from build123d import *

# Parameters (mm, degrees)
SKETCH1_W                                           = 107
SKETCH1_H                                           = 26
BOSS_EXTRUDE1_DEPTH                                 = 8
SKETCH2_W                                           = 1
SKETCH2_H                                           = 7.5
SKETCH2_W_2                                         = 6
SKETCH2_H_2                                         = 6.5
CUT_EXTRUDE1_DEPTH                                  = 111.403804282
FILLET1_R                                           = 0.5
CSK_FOR_M2_COUNTERSUNK_FLAT_HEAD_SCREW1_D           = 2.4
CSK_FOR_M2_COUNTERSUNK_FLAT_HEAD_SCREW1_DEPTH       = 15
CSK_FOR_M2_COUNTERSUNK_FLAT_HEAD_SCREW1_CSINK_D     = 4.4
CSK_FOR_M2_COUNTERSUNK_FLAT_HEAD_SCREW1_CSINK_ANGLE = 90
CSK_FOR_M2_COUNTERSUNK_FLAT_HEAD_SCREW1_TIP         = 0.721032743
SKETCH14_W                                          = 97
SKETCH14_H                                          = 24
CUT_EXTRUDE7_DEPTH                                  = 111.403804282
SKETCH14_3_W                                        = 97
SKETCH14_3_H                                        = 24
BOSS_EXTRUDE3_DEPTH                                 = 1
SKETCH18_W                                          = 97
SKETCH18_H                                          = 24
CUT_EXTRUDE8_DEPTH                                  = 111.403804282
SKETCH20_W                                          = 97
SKETCH20_H                                          = 24
SKETCH20_W_2                                        = 93
SKETCH20_H_2                                        = 20
BOSS_EXTRUDE4_DEPTH                                 = 8
SKETCH20_2_W                                        = 97
SKETCH20_2_H                                        = 24
SKETCH20_2_W_2                                      = 93
SKETCH20_2_H_2                                      = 20
CUT_EXTRUDE9_DEPTH                                  = 3
SKETCH21_W                                          = 52
SKETCH21_H                                          = 2
BOSS_EXTRUDE5_DEPTH                                 = 5
SKETCH22_W                                          = 52
SKETCH22_H                                          = 2
BOSS_EXTRUDE6_DEPTH                                 = 5
SKETCH23_W                                          = 0.5
SKETCH23_H                                          = 16.612240618
CUT_EXTRUDE10_DEPTH                                 = 111.403804282
BOSS_EXTRUDE7_REACH                                 = 111.249
SKETCH25_W                                          = 2
SKETCH25_H                                          = 5
CUT_EXTRUDE11_REACH                                 = 64.258
SKETCH26_W                                          = 10
SKETCH26_H                                          = 2
SKETCH27_W                                          = 97
SKETCH27_H                                          = 24
BOSS_EXTRUDE8_DEPTH                                 = 3
SKETCH29_W                                          = 20
SKETCH29_H                                          = 5
CUT_EXTRUDE12_DEPTH                                 = 54


with BuildPart() as part:
    # Sketch1 → Boss-Extrude1 (new body)
    with BuildSketch(Plane(origin=(0, 0, 0), x_dir=(1, 0, 0), z_dir=(0, 1, 0))):
        with Locations((53.5, -13)):
            Rectangle(SKETCH1_W, SKETCH1_H)
    extrude(amount=BOSS_EXTRUDE1_DEPTH)

    # Sketch2 → Cut-Extrude1 (cut, through all)
    with BuildSketch(Plane.XY.offset(26)):
        with Locations((106.5, 4.25)):
            Rectangle(SKETCH2_W, SKETCH2_H)
        with Locations((3, 4.75)):
            Rectangle(SKETCH2_W_2, SKETCH2_H_2)
    extrude(amount=-CUT_EXTRUDE1_DEPTH, mode=Mode.SUBTRACT)

    # Fillet1
    fillet1_edges = [part.edges().sort_by_distance(p)[0] for p in [
        (106, 8, 13),
        (0, 1.5, 13),
        (6, 8, 13),
    ]]
    fillet(fillet1_edges, radius=FILLET1_R)

    # CSK for M2 Countersunk Flat Head Screw1
    with Locations(Plane(origin=(3, 1.5, 13), x_dir=(1, 0, 0), z_dir=(0, 1, 0))):
        with Locations((0, 0)):
            CounterSinkHole(CSK_FOR_M2_COUNTERSUNK_FLAT_HEAD_SCREW1_D / 2, CSK_FOR_M2_COUNTERSUNK_FLAT_HEAD_SCREW1_CSINK_D / 2, depth=CSK_FOR_M2_COUNTERSUNK_FLAT_HEAD_SCREW1_DEPTH, counter_sink_angle=CSK_FOR_M2_COUNTERSUNK_FLAT_HEAD_SCREW1_CSINK_ANGLE)
            with Locations((0, 0, -(CSK_FOR_M2_COUNTERSUNK_FLAT_HEAD_SCREW1_DEPTH + CSK_FOR_M2_COUNTERSUNK_FLAT_HEAD_SCREW1_TIP / 2))):  # 118° drill point
                Cone(0, CSK_FOR_M2_COUNTERSUNK_FLAT_HEAD_SCREW1_D / 2, CSK_FOR_M2_COUNTERSUNK_FLAT_HEAD_SCREW1_TIP, mode=Mode.SUBTRACT)

    # Sketch14 → Cut-Extrude7 (cut, through all)
    with BuildSketch(Plane(origin=(0, 8, 0), x_dir=(1, 0, 0), z_dir=(0, 1, 0))):
        with Locations((56, -13)):
            Rectangle(SKETCH14_W, SKETCH14_H)
    extrude(amount=-CUT_EXTRUDE7_DEPTH, mode=Mode.SUBTRACT)

    # Sketch14<3> → Boss-Extrude3 (add)
    with BuildSketch(Plane(origin=(0, 8, 0), x_dir=(1, 0, 0), z_dir=(0, 1, 0))):
        with Locations((56, -13)):
            Rectangle(SKETCH14_3_W, SKETCH14_3_H)
    extrude(amount=-BOSS_EXTRUDE3_DEPTH)

    # Sketch18 → Cut-Extrude8 (cut, through all)
    with BuildSketch(Plane(origin=(0, 0, 0), x_dir=(1, 0, 0), z_dir=(0, 1, 0))):
        with Locations((56, -13)):
            Rectangle(SKETCH18_W, SKETCH18_H)
    extrude(amount=CUT_EXTRUDE8_DEPTH, mode=Mode.SUBTRACT)

    # Sketch20 → Boss-Extrude4 (add)
    with BuildSketch(Plane(origin=(0, 8, 0), x_dir=(1, 0, 0), z_dir=(0, 1, 0))):
        with Locations((56, -13)):
            Rectangle(SKETCH20_W, SKETCH20_H)
        with Locations((56, -13)):
            Rectangle(SKETCH20_W_2, SKETCH20_H_2, mode=Mode.SUBTRACT)
    extrude(amount=-BOSS_EXTRUDE4_DEPTH)

    # Sketch20<2> → Cut-Extrude9 (cut)
    with BuildSketch(Plane(origin=(0, 8, 0), x_dir=(1, 0, 0), z_dir=(0, 1, 0))):
        with Locations((56, -13)):
            Rectangle(SKETCH20_2_W, SKETCH20_2_H)
        with Locations((56, -13)):
            Rectangle(SKETCH20_2_W_2, SKETCH20_2_H_2, mode=Mode.SUBTRACT)
    extrude(amount=-CUT_EXTRUDE9_DEPTH, mode=Mode.SUBTRACT)

    # Sketch21 → Boss-Extrude5 (add)
    with BuildSketch(Plane.XY.offset(3)):
        with Locations((76.5, 1)):
            Rectangle(SKETCH21_W, SKETCH21_H)
    extrude(amount=BOSS_EXTRUDE5_DEPTH)

    # Sketch22 → Boss-Extrude6 (add)
    with BuildSketch(Plane(origin=(0, 0, 23), x_dir=(-1, 0, 0), z_dir=(0, 0, -1))):
        with Locations((-76.5, 1)):
            Rectangle(SKETCH22_W, SKETCH22_H)
    extrude(amount=BOSS_EXTRUDE6_DEPTH)

    # Sketch23 → Cut-Extrude10 (cut, through all)
    with BuildSketch(Plane.XY.offset(26)):
        with Locations((106.75, 8.306120309)):
            Rectangle(SKETCH23_W, SKETCH23_H)
    extrude(amount=-CUT_EXTRUDE10_DEPTH, mode=Mode.SUBTRACT)

    # Sketch25 → Boss-Extrude7 (add, up to next)
    with BuildSketch(Plane(origin=(0, 0, 23), x_dir=(-1, 0, 0), z_dir=(0, 0, -1)), mode=Mode.PRIVATE) as boss_extrude7_sk1:
        with Locations((-49.5, 2.5)):
            Rectangle(SKETCH25_W, SKETCH25_H)
    boss_extrude7_tool1 = extrude(boss_extrude7_sk1.sketch, amount=BOSS_EXTRUDE7_REACH, mode=Mode.PRIVATE) - part.part
    add(boss_extrude7_tool1.solids().sort_by_distance((49.5, 2.5, 23))[0])

    # Sketch26 → Cut-Extrude11 (cut, up to next)
    with BuildSketch(Plane(origin=(50.5, 0, 0), x_dir=(0, 0, -1), z_dir=(1, 0, 0)), mode=Mode.PRIVATE) as cut_extrude11_sk1:
        with Locations((-13, 1)):
            Rectangle(SKETCH26_W, SKETCH26_H)
    cut_extrude11_tool1 = extrude(cut_extrude11_sk1.sketch, amount=-CUT_EXTRUDE11_REACH, mode=Mode.PRIVATE) & part.part
    add(cut_extrude11_tool1.solids().sort_by_distance((50.5, 1, 13))[0], mode=Mode.SUBTRACT)

    # Sketch27 → Boss-Extrude8 (add)
    with BuildSketch(Plane(origin=(0, 5, 0), x_dir=(1, 0, 0), z_dir=(0, 1, 0))):
        with Locations((56, -13)):
            Rectangle(SKETCH27_W, SKETCH27_H)
    extrude(amount=BOSS_EXTRUDE8_DEPTH)

    # Sketch29 → Cut-Extrude12 (cut)
    with BuildSketch(Plane.ZY.offset(-48.5)):
        with Locations((13, 2.5)):
            Rectangle(SKETCH29_W, SKETCH29_H)
    extrude(amount=-CUT_EXTRUDE12_DEPTH, mode=Mode.SUBTRACT)


solid = part.part
Here's how the part is built. I have some questions about the finished solid (model axes, mm). A direction names the side the tool comes from. Round coordinates to 2 decimals unless told otherwise and drop trailing zeros. Order: outer loops, then holes, each group sorted by start corner. A loop starts at its lowest first (then second) coordinate and runs counter-clockwise, first axis right, second up. Notation, with made-up numbers: M 86.25,88.25 L 91.25,88.25 A14 ccw 91.25,111.25 Z; hole C 53,41.5 d11. An arc over 180 degrees is marked long. One line per question, with ' | ' between items.
1) We'd pull the mould along X, two halves only. Please class faces 4 (the flat face through (6, 4, 13)), 5 (the flat face through (50, 0, 2)), 6 (the flat face through (55, 5, 13)): released by +X, released by -X, zero draft, split by the parting line, or undercut.
Checked values:
face 4: released by -X | face 5: zero draft | face 6: undercut
2) I need wall thicknesses on line 1 (Z direction, x = 98, y = 4.75); line 2 (X direction, y = 4, z = 7); line 3 (X direction, y = 0.35, z = 13). Which ranges of each line are inside material? Lowest first, please.
Checked values:
line 1: z = 0 to 3, 23 to 26 | line 2: x = 6 to 9.5, 102.5 to 106 | line 3: x = 0 to 1.8, 4.2 to 9.5, 102.5 to 106.5
3) On a 3-axis mill with a long thin cutter (end or side, diameter ignored), from which of +Z, -Z, +X, -X, +Y, -Y can I reach the whole of each face in a straight line? I mean faces 1 (the flat face through (5.7, 1.5, 13.2)), 2 (the flat face through (9.5, 3, 13)), 3 (the flat face through (106, 4, 13)). Say none if no direction works.
Checked values:
face 1: +Z, -Z, -X, +Y | face 2: -Y | face 3: +Z, -Z, +X, +Y
4) Imagine slicing it at D-D, the plane x = 99. Write out the boundary of the cut face in (y, z), plus the area to 3 significant figures.
Checked values:
outline: M 0,0 L 8,0 L 8,26 L 0,26 L 0,23 L 5,23 L 5,3 L 0,3 Z | area: 108 mm²
5) Imagine slicing it at A-A, the plane z = 13. Write out the boundary of the cut face in (x, y).
Checked values:
outline: M 0,0 L 1.8,0 L 1.8,0.5 L 0.8,1.5 L 0.5,1.5 A0.5 ccw 0,1 Z; M 4.2,0 L 9.5,0 L 9.5,5 L 102.5,5 L 102.5,0 L 106.5,0 L 106.5,0.5 L 106,0.5 L 106,7.5 A0.5 ccw 105.5,8 L 6.5,8 A0.5 ccw 6,7.5 L 6,1.5 L 5.2,1.5 L 4.2,0.5 Z
6) Imagine slicing it at B-B, the plane x = 3. Write out the boundary of the cut face in (y, z), plus the area to 3 significant figures.
Checked values:
outline: M 0,0 L 1.5,0 L 1.5,10.8 L 0.5,11.8 L 0,11.8 Z; M 0,14.2 L 0.5,14.2 L 1.5,15.2 L 1.5,26 L 0,26 Z | area: 34.4 mm²
7) I'm going to push flat-ended pins straight in: pin 1 Ø4 at (y, z) = (1.5, 11) entering from -X; pin 2 Ø3.5 at (y, z) = (3, 7.5) entering from +X; pin 3 Ø2 at (y, z) = (6.5, 23.5) entering from -X; pin 4 Ø2 at (x, z) = (14.5, 10.5) entering from -Y. Where does each tip first touch, or does it pass through?
Checked values:
pin 1: stops at x = 0 | pin 2: stops at x = 106 | pin 3: stops at x = 6 | pin 4: stops at y = 5
8) Imagine slicing it at C-C, the plane z = 21.5. Write out the boundary of the cut face in (x, y), plus the area to 3 significant figures.
Checked values:
outline: M 0,0 L 9.5,0 L 9.5,5 L 102.5,5 L 102.5,0 L 106.5,0 L 106.5,0.5 L 106,0.5 L 106,7.5 A0.5 ccw 105.5,8 L 6.5,8 A0.5 ccw 6,7.5 L 6,1.5 L 0.5,1.5 A0.5 ccw 0,1 Z | area: 344 mm²
